```python
from build123d import *

# Parameters (mm, degrees)
SKETCH1_R                                            = 20
BOSS_EXTRUDE1_DEPTH                                  = 60.9
CBORE_FOR_M10_HEX_SOCKET_HEAD_CAP_SCREW1_D           = 10.5
CBORE_FOR_M10_HEX_SOCKET_HEAD_CAP_SCREW1_CBORE_D     = 18
CBORE_FOR_M10_HEX_SOCKET_HEAD_CAP_SCREW1_CBORE_DEPTH = 10.6
CHAMFER1_SIZE                                        = 2
CHAMFER2_SIZE                                        = 1
CHAMFER3_SIZE                                        = 1


with BuildPart() as part:
    # Sketch1 → Boss-Extrude1 (new body)
    with BuildSketch(Plane(origin=(0, 0, 0), x_dir=(1, 0, 0), z_dir=(0, 1, 0))):
        with Locations(Location((0, 0, 0), (0, 0, 270))):
            Circle(SKETCH1_R)
    extrude(amount=-BOSS_EXTRUDE1_DEPTH)

    # CBORE for M10 Hex Socket Head Cap Screw1 (through all)
    with Locations(Plane(origin=(0, 0, 0), x_dir=(1, 0, 0), z_dir=(0, 1, 0))):
        with Locations((0, 0)):
            CounterBoreHole(CBORE_FOR_M10_HEX_SOCKET_HEAD_CAP_SCREW1_D / 2, CBORE_FOR_M10_HEX_SOCKET_HEAD_CAP_SCREW1_CBORE_D / 2, CBORE_FOR_M10_HEX_SOCKET_HEAD_CAP_SCREW1_CBORE_DEPTH)

    # Chamfer1
    chamfer1_edges = [part.edges().sort_by_distance(p)[0] for p in [
        (0, 0, -20),
        (0, -60.9, -20),
    ]]
    chamfer(chamfer1_edges, length=CHAMFER1_SIZE)

    # Chamfer2
    chamfer2_edges = [part.edges().sort_by_distance(p)[0] for p in [
        (-9, 0, 0),
    ]]
    chamfer(chamfer2_edges, length=CHAMFER2_SIZE)

    # Chamfer3
    chamfer3_edges = [part.edges().sort_by_distance(p)[0] for p in [
        (5.25, -60.9, 0),
    ]]
    chamfer(chamfer3_edges, length=CHAMFER3_SIZE)


solid = part.part
```
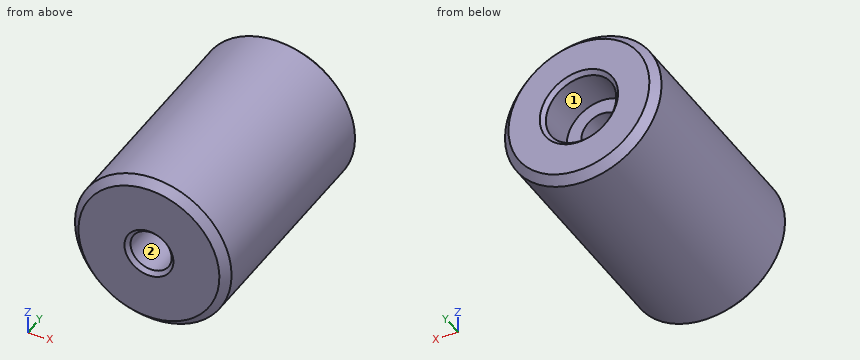
Could you check a few things on this model? Use its own coordinates, in mm. Face numbers are marked on the shaded views. A direction names the side the tool comes from. Coordinates: 2 decimals unless noted, no trailing zeros. Loops run counter-clockwise (first coordinate to the right, second up) from the corner with the lowest first, then second, coordinate; pieces in that order, holes last.
1) Which directions (+Z, -Z, +X, -X, +Y, -Y) give clear straight access to the entire face, cutting with the end or side of a thin tool? Please do the marked faces 1 and 2.
Reported:
face 1: +Y
face 2: +Y, -Y
2) Imagine slicing it at A-A (x = 0). List the corners of the cut face in (y, z) for me.
Reported:
outline: (-60.9, -18) - (-58.9, -20) - (-2, -20) - (0, -18) - (0, -10) - (-1, -9) - (-10.6, -9) - (-10.6, -5.25) - (-59.9, -5.25) - (-60.9, -6.25) - close; (-60.9, 6.25) - (-59.9, 5.25) - (-10.6, 5.25) - (-10.6, 9) - (-1, 9) - (0, 10) - (0, 18) - (-2, 20) - (-58.9, 20) - (-60.9, 18) - close
3) Please list where these lines run through material, in increasing order: line 1 along X through (y, z) = (-4.5, 0); line 2 along X through (y, z) = (-34, 0); line 3 along Z through (x, y) = (-2, -29).
Reported:
line 1: x = -20 to -9, 9 to 20
line 2: x = -20 to -5.25, 5.25 to 20
line 3: z = -19.9 to -4.85, 4.85 to 19.9
4) Will these pins go through, and if not, where does the flat tip stop? pin 1 Ø10 at (y, z) = (-38.5, -10) entering from -X; pin 2 Ø1 at (y, z) = (-23, 3.5) entering from +X; pin 3 Ø4 at (x, y) = (-7, -44.5) entering from +Z; pin 4 Ø6.5 at (x, z) = (0, 0) entering from -Y.
Reported:
pin 1: stops at x = -19.36
pin 2: stops at x = 19.77
pin 3: stops at z = 19.36
pin 4: passes through
5) Imagine slicing it at B-B (z = 0). List the corners of the cut face in (x, y) for me, and give its area (3 significant figures).
Reported:
outline: (-20, -58.9) - (-18, -60.9) - (-6.25, -60.9) - (-5.25, -59.9) - (-5.25, -10.6) - (-9, -10.6) - (-9, -1) - (-10, 0) - (-18, 0) - (-20, -2) - close; (5.25, -59.9) - (6.25, -60.9) - (18, -60.9) - (20, -58.9) - (20, -2) - (18, 0) - (10, 0) - (9, -1) - (9, -10.6) - (5.25, -10.6) - close
area: 1,710 mm2
